Model file for the job. Use its own axes, mm. A direction names the side the tool comes from. Round coordinates to 2 decimals unless told otherwise and drop trailing zeros. Loops run counter-clockwise (first coordinate to the right, second up) from the corner with the lowest first, then second, coordinate; pieces in that order, holes last. Notation, with made-up numbers: M -32,-9 L -23,-9 A12 ccw -23,-2 Z; hole C 53.5,-35 d11. An arc over 180 degrees is marked long. Use a Markdown table: item, result. Add a question column.
Item 1: Tool access for faces 1 (the flat face through (0, 840, 180)), 2 (the flat face through (0, 718, 45)), 3 (the flat face through (-82.555, 194.79, -61.342)): list every direction of +Z, -Z, +X, -X, +Y, -Y with a clear straight run to the whole face (end or side of a thin tool).
Item 2: Wall check: L1, parallel to Z at x = 2.5, y = 717; L2, parallel to Y at x = 3, z = 326 (3 decimals); L3, parallel to Z at x = 2.25, y = 757.5 (3 decimals). Give the ranges that are in metal, low to high. Write a range as from..to.
Item 3: Two-plate mould, pull along Y, no slides. Class faces 4 (the cylindrical face through (41.53, 44.37, 79.845)), 5 (the flat face through (-1, 0, -1)), 6 (the flat face through (-72, 180, -72)): +Y half, -Y half, draft (parallel to the pull), parting line (faces both ways), or undercut.
Item 4: Saw through at D-D on z = 27. Write the cut outline in (x, y).
Item 5: Pin check, flat tips, straight feed: P1, Ø10, axis at y = 682.5, z = 313.5, coming from the +X side; P2, Ø24, axis at x = 6.5, z = 161, coming from the +Y side; P3, Ø12, axis at y = 590.5, z = 160, coming from the +X side. Stop position of each tip, or through.
Item 6: Saw through at B-B on x = -25. Write the cut outline in (y, z).
Item 7: Saw through at C-C on z = 291. Write the cut outline in (x, y).
Item 8: Saw through at A-A on y = 625.5. Write the cut outline in (x, z).
```python
from build123d import *

# Parameters (mm, degrees)
SKETCH_1_R          = 90
EXTRUDE_1_DEPTH     = 90
SKETCH_2_W          = 30
SKETCH_2_H          = 30
EXTRUDE_2_DEPTH     = 970
SKETCH_3_W          = 30
SKETCH_3_H          = 30
EXTRUDE_3_DEPTH     = 200
SKETCH_5_W          = 400
SKETCH_5_H          = 300
SKETCH_5_W_2        = 340
SKETCH_5_H_2        = 240
EXTRUDE_5_DEPTH     = 30
SKETCH_7_W          = 130
SKETCH_7_H          = 240
SKETCH_7_R          = 3.175
EXTRUDE_6_DEPTH     = 30
SKETCH_8_W          = 130
SKETCH_8_H          = 240
CUT_EXTRUDE_1_DEPTH = 7
SKETCH_9_W          = 130
SKETCH_9_H          = 240
CUT_EXTRUDE_2_DEPTH = 7


with BuildPart() as part:
    # 草圖1 → 填料-伸長1 (new body)
    with BuildSketch(Plane(origin=(0, 0, 0), x_dir=(1, 0, 0), z_dir=(0, 1, 0))):
        Circle(SKETCH_1_R)
    extrude(amount=EXTRUDE_1_DEPTH)

    # 草圖2 → 填料-伸長2 (add)
    with BuildSketch(Plane(origin=(0, 90, 0), x_dir=(1, 0, 0), z_dir=(0, 1, 0))):
        Rectangle(SKETCH_2_W, SKETCH_2_H)
    extrude(amount=EXTRUDE_2_DEPTH)

    # 草圖3 → 填料-伸長3 (add)
    with BuildSketch(Plane(origin=(0, 0, 0), x_dir=(-0.707106781, 0, 0.707106781), z_dir=(-0.707106781, 0, -0.707106781))):
        with Locations((0, 195)):
            Rectangle(SKETCH_3_W, SKETCH_3_H)
    extrude(amount=EXTRUDE_3_DEPTH)

    # 草圖5 → 填料-伸長5 (add)
    with BuildSketch(Plane(origin=(15, 0, 0), x_dir=(0, 0, -1), z_dir=(1, 0, 0))):
        with Locations((-215, 720)):
            Rectangle(SKETCH_5_W, SKETCH_5_H)
        with Locations((-215, 720)):
            Rectangle(SKETCH_5_W_2, SKETCH_5_H_2, mode=Mode.SUBTRACT)
    extrude(amount=-EXTRUDE_5_DEPTH)

    # 草圖7 → 填料-伸長6 (add)
    with BuildSketch(Plane.ZY.offset(15)):
        with Locations((276, 720)):
            Rectangle(SKETCH_7_W, SKETCH_7_H)
        with Locations((313.5, 757.5)):
            Circle(SKETCH_7_R, mode=Mode.SUBTRACT)
        with Locations((238.5, 757.5)):
            Circle(SKETCH_7_R, mode=Mode.SUBTRACT)
        with Locations((238.5, 682.5)):
            Circle(SKETCH_7_R, mode=Mode.SUBTRACT)
        with Locations((313.5, 682.5)):
            Circle(SKETCH_7_R, mode=Mode.SUBTRACT)
        with Locations((326, 770)):
            Circle(SKETCH_7_R, mode=Mode.SUBTRACT)
        with Locations((226, 770)):
            Circle(SKETCH_7_R, mode=Mode.SUBTRACT)
        with Locations((326, 670)):
            Circle(SKETCH_7_R, mode=Mode.SUBTRACT)
        with Locations((226, 670)):
            Circle(SKETCH_7_R, mode=Mode.SUBTRACT)
    extrude(amount=-EXTRUDE_6_DEPTH)

    # 草圖8 → 除料-伸長1 (cut)
    with BuildSketch(Plane.ZY.offset(15)):
        with Locations((276, 720)):
            Rectangle(SKETCH_8_W, SKETCH_8_H)
    extrude(amount=-CUT_EXTRUDE_1_DEPTH, mode=Mode.SUBTRACT)

    # 草圖9 → 除料-伸長2 (cut)
    with BuildSketch(Plane(origin=(15, 0, 0), x_dir=(0, 0, -1), z_dir=(1, 0, 0))):
        with Locations((-276, 720)):
            Rectangle(SKETCH_9_W, SKETCH_9_H)
    extrude(amount=-CUT_EXTRUDE_2_DEPTH, mode=Mode.SUBTRACT)


solid = part.part
```
Entries:
| question | item | result |
|---|---|---|
| 1 | face 1 | none |
| 1 | face 2 | +X, -X |
| 1 | face 3 | +Z, -X, +Y |
| 2 | L1 | -15..45, 211..341, 385..415 |
| 2 | L2 | 570..666.825, 673.175..766.825, 773.175..870 |
| 2 | L3 | -15..45, 211..235.325, 241.675..310.325, 316.675..341, 385..415 |
| 3 | face 4 | draft |
| 3 | face 5 | -Y half |
| 3 | face 6 | undercut |
| 4 | outline | M -85.85,0 L 85.85,0 L 85.85,90 L -85.85,90 Z; M -15,570 L 15,570 L 15,870 L -15,870 Z |
| 5 | P1 | x = 8 |
| 5 | P2 | y = 870 |
| 5 | P3 | x = 15 |
| 6 | outline | M 0,-86.46 L 90,-86.46 L 90,86.46 L 0,86.46 Z; M 180,-46.21 L 210,-46.21 L 210,-3.79 L 180,-3.79 Z |
| 7 | outline | M -15,570 L 15,570 L 15,600 L 8,600 L 8,840 L 15,840 L 15,870 L -15,870 L -15,840 L -8,840 L -8,600 L -15,600 Z |
| 8 | outline | M -15,-15 L 15,-15 L 15,45 L -15,45 Z; M -15,385 L 15,385 L 15,415 L -15,415 Z; M -8,211 L 8,211 L 8,341 L -8,341 Z |
